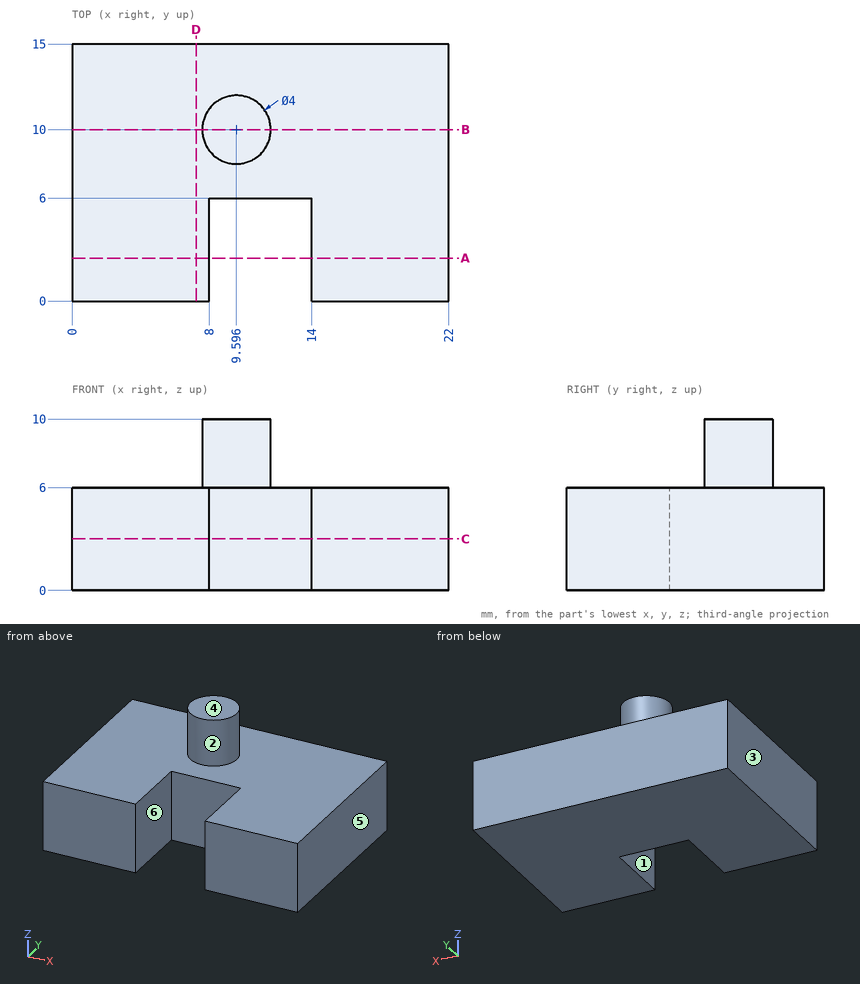
Design review of the part shown in the three views and the two pictorial views. Dimensions are in mm from the part's minimum x, y and z. A direction names the side the tool comes from. Round coordinates to 2 decimals unless told otherwise and drop trailing zeros. Order: outer loops, then holes, each group sorted by start corner. A loop starts at its lowest first (then second) coordinate and runs counter-clockwise, first axis right, second up.
(1) Mouldability with a two-part tool opening along X and no side actions: class the marked faces 1, 2, 3 and 4 as released by +X, released by -X, zero draft, split by the parting line, or undercut.
Working result:
face 1: undercut
face 2: split by the parting line
face 3: released by -X
face 4: zero draft
(2) Wall thickness on L1, parallel to Z at x = 3.25, y = 10.75; L2, parallel to X at y = 11, z = 8.5; L3, parallel to X at y = 9.5, z = 6.25: over which ranges is each line inside the solid? List them lowest first.
Working result:
L1: z = 0 to 6
L2: x = 7.86 to 11.33
L3: x = 7.66 to 11.53
(3) Take a section at D-D, the plane x = 7.25. State the section outline as (y, z) points, plus the area to 3 significant figures.
Working result:
outline: (0, 0) - (15, 0) - (15, 6) - (0, 6) - close
area: 90.0 mm2
(4) Take a section at A-A, the plane y = 2.5. State the section outline as (x, z) points.
Working result:
outline: (0, 0) - (8, 0) - (8, 6) - (0, 6) - close; (14, 0) - (22, 0) - (22, 6) - (14, 6) - close
(5) Tool access review of the marked faces 5 and 6: name each direction out of +Z, -Z, +X, -X, +Y, -Y from which nothing blocks a thin tool from reaching the whole face with its end or side.
Working result:
face 5: +Z, -Z, +X, +Y, -Y
face 6: +Z, -Z, -Y
(6) For P1, Ø3, axis at x = 11, y = 3, coming from the -Z side, flat-tipped, find the tip position at first contact; note if it passes through.
Working result:
P1: passes through
(7) Take a section at C-C, the plane z = 3. State the section outline as (x, y) points, plus the area to 3 significant figures.
Working result:
outline: (0, 0) - (8, 0) - (8, 6) - (14, 6) - (14, 0) - (22, 0) - (22, 15) - (0, 15) - close
area: 294 mm2
(8) Take a section at B-B, the plane y = 10. State the section outline as (x, z) points.
Working result:
outline: (0, 0) - (22, 0) - (22, 6) - (11.6, 6) - (11.6, 10) - (7.6, 10) - (7.6, 6) - (0, 6) - close
